from build123d import *

# Parameters (mm, degrees)
F0_W     = 59.02
F0_H     = 20.92
F0_W_2   = 48.86
F0_H_2   = 10.76
F1_DEPTH = 24.4475
F2_W     = 59.02
F2_H     = 7.62
F2_R     = 2.6035
F3_DEPTH = 5.08
F5_DEPTH = 24.4485
F6_W     = 48.86
F6_H     = 10.76
F7_DEPTH = 1.5875


with BuildPart() as f1:
    # F0 (on Top) → F1 (new body)
    with BuildSketch(Plane.XY):
        Rectangle(F0_W, F0_H)
        Rectangle(F0_W_2, F0_H_2, mode=Mode.SUBTRACT)
    extrude(amount=F1_DEPTH)

    # F2 (on face) → F3 (join)
    with BuildSketch(Plane.XY.offset(24.4475)):
        with Locations((0, 14.27)):
            Rectangle(F2_W, F2_H)
        with Locations((0, 13.635)):
            Circle(F2_R, mode=Mode.SUBTRACT)
    extrude(amount=-F3_DEPTH)

    # F4 (on face) → F5 (cut, through all)
    with BuildSketch(Plane(origin=(0, 0, 0), x_dir=(1, 0, 0), z_dir=(0, 0, -1))):
        Polygon((24.43, 5.38), (29.51, 5.38), (29.51, 10.46), (-29.51, 10.46), (-29.51, 5.38), (-24.43, 5.38), align=None)
    extrude(amount=-F5_DEPTH, mode=Mode.SUBTRACT)

    # F6 (on face) → F7 (join)
    with BuildSketch(Plane.XY.offset(24.4475)):
        Rectangle(F6_W, F6_H)
    extrude(amount=-F7_DEPTH)


solid = f1.part
The model under review builds one solid part; all positions refer to its coordinate system, in mm. A direction names the side the tool comes from. Give positions to 0.01 mm unless a question says otherwise; leave off trailing zeros. Write each loop counter-clockwise with the first axis right and the second up, starting at its lowest first coordinate (ties: lowest second). Pieces come first, ordered by that corner, then holes.
1. Tool access review of faces 5 (the flat face through (0, 0, 22.86)), 6 (the flat face through (29.51, 4, 12)), 7 (the flat face through (0, 17, 19.368)): name each direction out of +Z, -Z, +X, -X, +Y, -Y from which nothing blocks a thin tool from reaching the whole face with its end or side.
2. Add section B-B, the plane z = 5.75. Write out the cut boundary in (x, y).
3. For P1, Ø4, axis at x = 1, z = 13.5, coming from the +Y side; P2, Ø3, axis at x = 3, z = 12, coming from the -Y side; P3, Ø6, axis at x = 1.5, y = 14, coming from the -Z side, all flat-tipped, find the tip position at first contact; note any pin that passes through.
4. Add section A-A, the plane x = 0. Write out the cut boundary in (y, z), plus the area to 3 significant figures.
5. Wall thickness on L1, parallel to X at y = 4.75, z = 15.25; L2, parallel to Y at x = 0, z = 22.2; L3, parallel to Z at x = 3, y = 16: over which ranges is each line inside the solid? List them lowest first.
6. Add section C-C, the plane y = 0.25. Write out the cut boundary in (x, z).
7. Draft analysis for pull direction Y (two halves, no side actions). For faces 1 (the flat face through (0, -5.38, 24)), 2 (the flat face through (24.43, 0, 11)), 3 (the cylindrical face through (1.4, 15.83, 21.94)), 4 (the flat face through (0, 10.46, 10)), state which applies: +Y half, -Y half, draft (parallel to the pull), parting line (faces both ways), or undercut.
Worked answers:
1. face 5: -Z, -Y
1. face 6: +Z, -Z, +X, +Y, -Y
1. face 7: -Z, +X, -X, +Y
2. outline: (-29.51, -5.38) - (-24.43, -5.38) - (-24.43, 5.38) - (24.43, 5.38) - (24.43, -5.38) - (29.51, -5.38) - (29.51, 10.46) - (-29.51, 10.46) - close
3. P1: stops at y = 10.46
3. P2: stops at y = 5.38
3. P3: stops at z = 19.37
4. outline: (-5.38, 22.86) - (5.38, 22.86) - (5.38, 0) - (10.46, 0) - (10.46, 19.37) - (11.03, 19.37) - (11.03, 24.45) - (-5.38, 24.45) - close; (16.24, 19.37) - (18.08, 19.37) - (18.08, 24.45) - (16.24, 24.45) - close
4. area: 154 mm2
5. L1: x = -29.51 to -24.43, 24.43 to 29.51
5. L2: y = 5.38 to 11.03, 16.24 to 18.08
5. L3: z = 19.37 to 24.45
6. outline: (-29.51, 0) - (-24.43, 0) - (-24.43, 22.86) - (24.43, 22.86) - (24.43, 0) - (29.51, 0) - (29.51, 24.45) - (-29.51, 24.45) - close
7. face 1: -Y half
7. face 2: draft
7. face 3: undercut
7. face 4: +Y half
